Could you check a few things on this drawing? It's one solid part, dimensions in mm from its lowest x, y, z. A direction names the side the tool comes from. Round coordinates to 2 decimals unless told otherwise and drop trailing zeros. Order: outer loops, then holes, each group sorted by start corner. A loop starts at its lowest first (then second) coordinate and runs counter-clockwise, first axis right, second up.
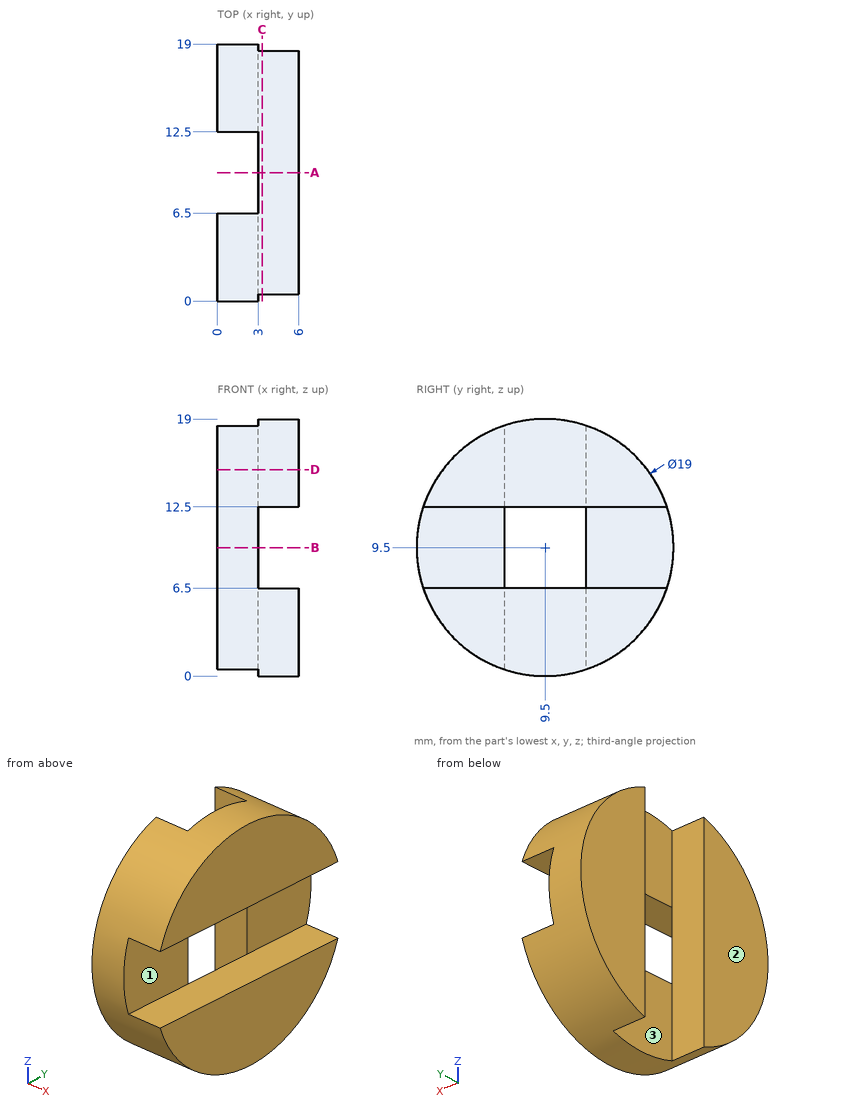
(1) I want a section at A-A, the plane y = 9.5. List the corners of the cut face in (x, z) for me, plus the area to 3 significant figures.
(2) I'm going to push flat-ended pins straight in: pin 1 Ø2.5 at (x, y) = (5, 12.5) entering from +Z; pin 2 Ø2.5 at (x, z) = (1, 7.5) entering from -Y; pin 3 Ø2 at (x, z) = (2.5, 14.5) entering from -Y. Where does each tip first touch, or does it pass through?
(3) I want a section at D-D, the plane z = 15.25. List the corners of the cut face in (x, y) for me, plus the area to 3 significant figures.
(4) Please list where these lines run through material, in increasing order: probe 1 along X at (y, z) = (17.75, 7.25); probe 2 along Z at (x, y) = (4.85, 15.75); probe 3 along Y at (x, z) = (1.5, 6.75).
(5) On a 3-axis mill with a long thin cutter (end or side, diameter ignored), from which of +Z, -Z, +X, -X, +Y, -Y can I reach the whole of each face in a straight line? I mean the marked faces 1, 2 and 3. Say none if no direction works.
(6) I want a section at B-B, the plane z = 9.5. List the corners of the cut face in (x, y) for me.
(7) I want a section at C-C, the plane x = 3.3. List the corners of the cut face in (y, z) for me.
Ans:
1. outline: (3, 0) - (6, 0) - (6, 6.5) - (3, 6.5) - close; (3, 12.5) - (6, 12.5) - (6, 19) - (3, 19) - close
1. area: 39.0 mm2
2. pin 1: stops at z = 18.84
2. pin 2: stops at y = 0.03
2. pin 3: stops at y = 0.88
3. outline: (0, 1.94) - (6, 1.94) - (6, 17.06) - (0, 17.06) - (0, 12.5) - (3, 12.5) - (3, 6.5) - (0, 6.5) - close
3. area: 72.7 mm2
4. probe 1: x = 0 to 3
4. probe 2: z = 2.35 to 6.5, 12.5 to 16.65
4. probe 3: y = 0.41 to 6.5, 12.5 to 18.59
5. face 1: +X, +Y, -Y
5. face 2: +Z, -Z, -X, +Y, -Y
5. face 3: +Z, -Z, -X
6. outline: (0, 0) - (3, 0) - (3, 6.5) - (0, 6.5) - close; (0, 12.5) - (3, 12.5) - (3, 19) - (0, 19) - close
7. outline: (0.49, 6.5) arc R9.5 ccw to (18.51, 6.5) - close; (0.49, 12.5) - (18.51, 12.5) arc R9.5 ccw to start
